```python
from build123d import *

# Parameters (mm, degrees)
F0_W       = 76.2
F0_H       = 69.85
F1_DEPTH   = 63.5
F2_W       = 38.1
F2_H       = 6.35
F3_DEPTH   = 76.201
F4_W       = 63.5
F4_H       = 19.05
F5_DEPTH   = 63.501
F6_W       = 63.5
F6_H       = 38.1
F7_DEPTH   = 63.501
F8_W       = 31.75
F8_H       = 7.874
F9_DEPTH   = 25.4
F11_DEPTH  = 25.4
F12_W      = 38.1
F12_H      = 15.748
F13_DEPTH  = 12.701
F14_R      = 12.7
F14_R_2    = 7.112
F15_DEPTH  = 4.064
F15_FACE_R = 7.112
F16_DEPTH  = 31.751


with BuildPart() as f1:
    # F0 (on Front) → F1 (new body)
    with BuildSketch(Plane.XZ):
        with Locations((38.1, 34.925)):
            Rectangle(F0_W, F0_H)
    extrude(amount=F1_DEPTH)

    # F2 (on face) → F3 (cut, through all)
    with BuildSketch(Plane.YZ.offset(76.2)):
        with Locations((-31.75, 3.175)):
            Rectangle(F2_W, F2_H)
    extrude(amount=-F3_DEPTH, mode=Mode.SUBTRACT)

    # F4 (on face) → F5 (cut, through all)
    with BuildSketch(Plane.XZ.offset(63.5)):
        with Locations((31.75, 9.525)):
            Rectangle(F4_W, F4_H)
    extrude(amount=-F5_DEPTH, mode=Mode.SUBTRACT)

    # F6 (on face) → F7 (cut, through all)
    with BuildSketch(Plane.XZ.offset(63.5)):
        with Locations((44.45, 50.8)):
            Rectangle(F6_W, F6_H)
    extrude(amount=-F7_DEPTH, mode=Mode.SUBTRACT)

    # F8 (on face) → F9 (cut)
    with BuildSketch(Plane.XY.offset(31.75)):
        with Locations((44.323, -59.563)):
            Rectangle(F8_W, F8_H)
        with Locations((44.323, -3.937)):
            Rectangle(F8_W, F8_H)
    extrude(amount=-F9_DEPTH, mode=Mode.SUBTRACT)

    # F10 (on face) → F11 (cut)
    with BuildSketch(Plane.YZ.offset(12.7)):
        with BuildLine():
            ThreePointArc((-63.5, 57.15), (-59.780256, 66.130256), (-50.8, 69.85))
            Line((-50.8, 69.85), (-63.5, 69.85))
            Line((-63.5, 69.85), (-63.5, 57.15))
        make_face()
        with BuildLine():
            Line((0, 69.85), (-12.7, 69.85))
            ThreePointArc((-12.7, 69.85), (-3.719744, 66.130256), (0, 57.15))
            Line((0, 57.15), (0, 69.85))
        make_face()
    extrude(amount=-F11_DEPTH, mode=Mode.SUBTRACT)

    # F12 (on face) → F13 (cut, through all)
    with BuildSketch(Plane.YZ.offset(12.7)):
        with Locations((-31.75, 54.102)):
            Rectangle(F12_W, F12_H)
        with BuildLine():
            Line((-50.8, 46.228), (-50.8, 61.976))
            ThreePointArc((-50.8, 61.976), (-58.674, 54.102), (-50.8, 46.228))
        make_face()
        with BuildLine():
            ThreePointArc((-12.7, 46.228), (-4.826, 54.102), (-12.7, 61.976))
            Line((-12.7, 61.976), (-12.7, 46.228))
        make_face()
    extrude(amount=-F13_DEPTH, mode=Mode.SUBTRACT)

    # F14 (on face) → F15 (cut)
    with BuildSketch(Plane.XY.offset(31.75)):
        with Locations((44.45, -31.75)):
            Circle(F14_R)
        with Locations((44.45, -31.75)):
            Circle(F14_R_2, mode=Mode.SUBTRACT)
    extrude(amount=-F15_DEPTH, mode=Mode.SUBTRACT)

    # F15_face (on face) → F16 (cut, through all)
    with BuildSketch(Plane(origin=(44.45, -31.75, 31.75), x_dir=(1, 0, 0), z_dir=(0, 0, 1))):
        Circle(F15_FACE_R)
    extrude(amount=-F16_DEPTH, mode=Mode.SUBTRACT)


solid = f1.part
```
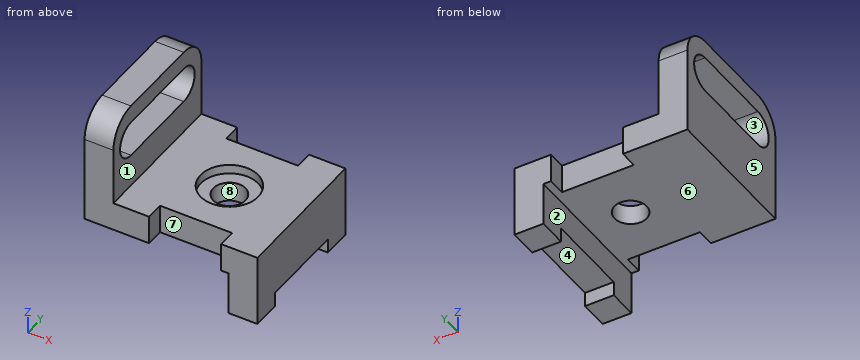
Here's how the part is built. I have some questions about the finished solid (model axes, mm). Face numbers are marked on the shaded views. A direction names the side the tool comes from. Coordinates: 2 decimals unless noted, no trailing zeros. Loops run counter-clockwise (first coordinate to the right, second up) from the corner with the lowest first, then second, coordinate; pieces in that order, holes last. Notation, with made-up numbers: M 44,29 L 93,29 A15 cw 93,36 Z; hole C 40,-38 d2. An arc over 180 degrees is marked long. One line per item, written item: value.
1. Please list where these lines run through material, in increasing order: probe 1 along Y at (x, z) = (44.45, 28.7); probe 2 along X at (y, z) = (-31, 29); probe 3 along Y at (x, z) = (44, 23).
Geometry says:
probe 1: y = -55.63 to -44.45, -19.05 to -7.87
probe 2: x = 0 to 31.77, 57.13 to 76.2
probe 3: y = -55.63 to -38.85, -24.65 to -7.87
2. Imagine slicing it at A-A (y = -31.75). List the corners of the cut face in (x, z) for me.
Geometry says:
outline: M 0,19.05 L 37.34,19.05 L 37.34,27.69 L 31.75,27.69 L 31.75,31.75 L 12.7,31.75 L 12.7,46.23 L 0,46.23 Z; M 0,61.98 L 12.7,61.98 L 12.7,69.85 L 0,69.85 Z; M 51.56,19.05 L 63.5,19.05 L 63.5,6.35 L 76.2,6.35 L 76.2,31.75 L 57.15,31.75 L 57.15,27.69 L 51.56,27.69 Z
3. Imagine slicing it at B-B (x = 44.45). List the corners of the cut face in (y, z) for me, and give its area (3 significant figures).
Geometry says:
outline: M -55.63,19.05 L -38.86,19.05 L -38.86,27.69 L -44.45,27.69 L -44.45,31.75 L -55.63,31.75 Z; M -24.64,19.05 L -7.87,19.05 L -7.87,31.75 L -19.05,31.75 L -19.05,27.69 L -24.64,27.69 Z
area: 380 mm2
4. Will these pins go through, and if not, where does the flat tip stop? pin 1 Ø8 at (x, y) = (61, -35) entering from +Z; pin 2 Ø7.5 at (x, y) = (50.5, -36) entering from +Z; pin 3 Ø10 at (x, y) = (7.5, -29.5) entering from -Z.
Geometry says:
pin 1: stops at z = 31.75
pin 2: stops at z = 27.69
pin 3: stops at z = 19.05
5. Thinking about a two-plate mould opening in X: for the marked faces 5, 6, 7 and 8, which applies, +X half, -X half, draft (parallel to the pull), parting line (faces both ways), or undercut?
Geometry says:
face 5: -X half
face 6: draft
face 7: undercut
face 8: undercut
6. Imagine slicing it at C-C (z = 55). List the corners of the cut face in (x, y) for me.
Geometry says:
outline: M 0,-63.5 L 12.7,-63.5 L 12.7,-58.62 L 0,-58.62 Z; M 0,-4.88 L 12.7,-4.88 L 12.7,0 L 0,0 Z
7. On a 3-axis mill with a long thin cutter (end or side, diameter ignored), from which of +Z, -Z, +X, -X, +Y, -Y can I reach the whole of each face in a straight line? I mean the marked faces 1, 2, 3 and 4. Say none if no direction works.
Geometry says:
face 1: +Z, +X, +Y, -Y
face 2: -Z, -X, +Y, -Y
face 3: +X, -X
face 4: -Z, +X, -X
8. Imagine slicing it at D-D (x = 71). List the corners of the cut face in (y, z) for me.
Geometry says:
outline: M -63.5,0 L -50.8,0 L -50.8,6.35 L -12.7,6.35 L -12.7,0 L 0,0 L 0,31.75 L -63.5,31.75 Z
